from build123d import *

# Parameters (mm, degrees)
F1_DEPTH = 40
F2_R     = 1.5
F3_DEPTH = 25
F4_R     = 1.5
F5_DEPTH = 7


with BuildPart() as f1:
    # F0 (on Front) → F1 (new body)
    with BuildSketch(Plane.XZ):
        Polygon((0, 0), (0, 7.5), (-6, 7.5), (-6, 8.5), (-6.5, 8.5), (-6.5, 0), align=None)
        Polygon((6, 7.5), (0, 7.5), (0, 0), (6.5, 0), (6.5, 8.5), (6, 8.5), align=None)
    extrude(amount=F1_DEPTH)

    # F2 (on face) → F3 (cut)
    with BuildSketch(Plane.XY.offset(7.5)):
        with Locations((0, -20)):
            Circle(F2_R)
    extrude(amount=-F3_DEPTH, mode=Mode.SUBTRACT)

    # F4 (on face) → F5 (cut)
    with BuildSketch(Plane.XZ.offset(40)):
        with Locations((-3, 3.75)):
            Circle(F4_R)
        with Locations((3, 3.75)):
            Circle(F4_R)
    extrude(amount=-F5_DEPTH, mode=Mode.SUBTRACT)


solid = f1.part
Build history of the part. All positions in model axes, mm. A direction names the side the tool comes from. Round coordinates to 2 decimals unless told otherwise and drop trailing zeros. Loops run counter-clockwise (first coordinate to the right, second up) from the corner with the lowest first, then second, coordinate; pieces in that order, holes last. Notation, with made-up numbers: (67, 5) -> (89, 5) arc R32 ccw to (89, 44) -> close; hole circle Ø9 at (83, -24.5). An arc over 180 degrees is marked (long way). Use CSV: the item, a comma, the result in double quotes. Start each with the question number.
Q1. Saw through at D-D on y = -4.5. Give the cut face in (x, z).
Q2. Saw through at C-C on y = -19.5. Give the cut face in (x, z), and give its area (3 significant figures).
Q3. Flat gauge pins, fed straight in: pin 1 Ø1.5 at (x, z) = (-2.5, 4) entering from -Y; pin 2 Ø3 at (x, y) = (0, -4) entering from +Z. Where does each tip first touch, or does it go through?
Q4. Drill centre lines: L1, parallel to X at y = -19, z = 8; L2, parallel to Y at x = 0, z = 4.75; L3, parallel to Z at x = -3, y = -34.75. Where is each one in solid material? Low to high.
Q5. Saw through at A-A on x = 0. Give the cut face in (y, z).
Q6. Mould opens along Z. For faces 1 (the face through (3, -33, 4)), 2 (the face through (-3, -20, 7.5)), 3 (the face through (0, 0, 4)) say: +Z half, -Z half, draft (parallel to the pull), parting line (faces both ways), or undercut.
Q7. Saw through at B-B on z = 3.75. Give the cut face in (x, y), and give its area (3 significant figures).
Q8. Which spindle directions (+Z, -Z, +X, -X, +Y, -Y) get a long thin tool onto all of the face, cutting with end or side? Do faces 4 (the face through (0, -40, 4)), 5 (the face through (4.386, -36.549, 3.175)), 6 (the face through (-6, -20, 8)). Say none if no direction does.
Solutions:
1,outline,"(-6.5, 0) -> (6.5, 0) -> (6.5, 8.5) -> (6, 8.5) -> (6, 7.5) -> (-6, 7.5) -> (-6, 8.5) -> (-6.5, 8.5) -> close"
2,outline,"(-6.5, 0) -> (-1.41, 0) -> (-1.41, 7.5) -> (-6, 7.5) -> (-6, 8.5) -> (-6.5, 8.5) -> close; (1.41, 0) -> (6.5, 0) -> (6.5, 8.5) -> (6, 8.5) -> (6, 7.5) -> (1.41, 7.5) -> close"
2,area,"77.3 mm^2"
3,pin 1,"stops at y = -33"
3,pin 2,"stops at z = 7.5"
4,L1,"x = -6.5 to -6, 6 to 6.5"
4,L2,"y = -40 to -21.5, -18.5 to 0"
4,L3,"z = 0 to 2.25, 5.25 to 7.5"
5,outline,"(-40, 0) -> (-21.5, 0) -> (-21.5, 7.5) -> (-40, 7.5) -> close; (-18.5, 0) -> (0, 0) -> (0, 7.5) -> (-18.5, 7.5) -> close"
6,face 1,"undercut"
6,face 2,"+Z half"
6,face 3,"draft"
7,outline,"(-6.5, -40) -> (-4.5, -40) -> (-4.5, -33) -> (-1.5, -33) -> (-1.5, -40) -> (1.5, -40) -> (1.5, -33) -> (4.5, -33) -> (4.5, -40) -> (6.5, -40) -> (6.5, 0) -> (-6.5, 0) -> close; hole circle Ø3 at (0, -20)"
7,area,"471 mm^2"
8,face 4,"+Z, -Z, +X, -X, -Y"
8,face 5,"-Y"
8,face 6,"+Z, +Y, -Y"
